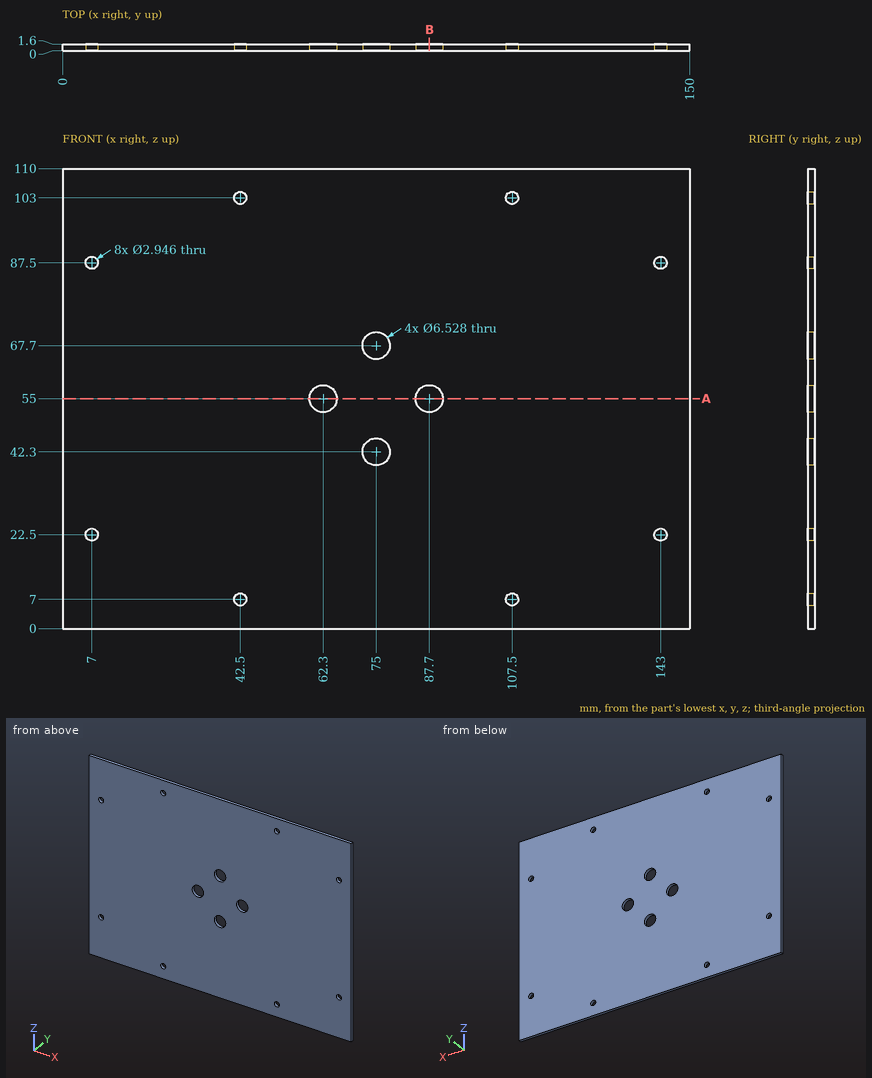
For this review, use the dimensioned drawing (mm, ordinates from the lowest corner) and the shaded views. Round coordinates to 2 decimals unless told otherwise and drop trailing zeros. Order: outer loops, then holes, each group sorted by start corner. A loop starts at its lowest first (then second) coordinate and runs counter-clockwise, first axis right, second up. Notation, with made-up numbers: M 75,-18.5 L 113,-18.5 A33 ccw 113,17.5 Z; hole C 21,10 d8. An arc over 180 degrees is marked long. Use a Markdown table: item, result. Add a question column.
Item 1: Add section B-B, the plane x = 87.7. Give the boundary of the cut face in (y, z).
Item 2: To check wall thickness, follow line 1 along X through (y, z) = (0.4, 22.5); line 2 along Z through (x, y) = (142.5, 0.4) (1 decimal); line 3 along X through (y, z) = (0.55, 42.3). State the ranges of each line that lie inside material, in increasing order.
Item 3: Add section A-A, the plane z = 55. Give the boundary of the cut face in (x, y).
Geometry results:
| question | item | result |
|---|---|---|
| 1 | outline | M 0,0 L 1.6,0 L 1.6,51.74 L 0,51.74 Z; M 0,58.26 L 1.6,58.26 L 1.6,110 L 0,110 Z |
| 2 | line 1 | x = 0 to 5.53, 8.47 to 141.53, 144.47 to 150 |
| 2 | line 2 | z = 0 to 21.1, 23.9 to 86.1, 88.9 to 110 |
| 2 | line 3 | x = 0 to 71.74, 78.26 to 150 |
| 3 | outline | M 0,0 L 59.04,0 L 59.04,1.6 L 0,1.6 Z; M 65.56,0 L 84.44,0 L 84.44,1.6 L 65.56,1.6 Z; M 90.96,0 L 150,0 L 150,1.6 L 90.96,1.6 Z |
